Design review of the part built by this model. Coordinates are the model's own, in mm. A direction names the side the tool comes from. Give positions to 0.01 mm unless a question says otherwise; leave off trailing zeros. Write each loop counter-clockwise with the first axis right and the second up, starting at its lowest first coordinate (ties: lowest second). Pieces come first, ordered by that corner, then holes. Notation, with made-up numbers: (84.25, 13.5) -> (126.25, 13.5) arc R34 cw to (126.25, 44.5) -> close; hole circle Ø11 at (80.25, 22.5). An arc over 180 degrees is marked (long way). Write each question's results on one line, items separated by ' | '. Start each with the question number.
(1) Take a section at B-B (x = 0). State the section outline as (y, z) points, plus the area to 3 significant figures.
(2) Take a section at A-A (y = 41). State the section outline as (x, z) points.
(3) Take a section at D-D (x = -21). State the section outline as (y, z) points.
(4) Clearance check with flat-ended pins moving along their axes: pin 1 (3.5 mm diameter, centred on y = 43, z = 3, fed in from -X); pin 2 (2 mm diameter, centred on y = 9.5, z = 4.5, fed in from +X); pin 3 (3.5 mm diameter, centred on x = -5, z = 2, fed in from +Y); pin 4 (3 mm diameter, centred on y = 44.6, z = 3.5, fed in from +X). State where each tip first meets the part, or that it passes through.
(5) Take a section at C-C (z = 3.5). Count the separate pieces of the cut face and the enclosed holes in it, plus the area to 3 significant figures.
(6) For faces 5 (the face through (0, 29, 7)), 6 (the face through (5, 12, 3)), 7 (the face through (0, 34.6, 3)), 8 (the face through (-5, 13, 3)), list the 3-axis set-ups (+Z, -Z, +X, -X, +Y, -Y) from which the entire face can be reached by the end or side of a thin tool; tool diameter is ignored.
(7) Mouldability with a two-part tool opening along X and no side actions: class faces 1 (the face through (-3.924, -3.954, 3.451)), 2 (the face through (-20.1, 42, 3)), 3 (the face through (20.1, 47, 3)), 4 (the face through (0, -5, 3)) as released by +X, released by -X, zero draft, split by the parting line, or undercut.
(8) To check wall thickness, follow probe 1 along X at (y, z) = (40.5, 6); probe 2 along Y at (x, z) = (-17.5, 0.75); probe 3 along X at (y, z) = (51, 6). State the ranges of each line that lie inside material, in increasing order.
from build123d import *

# Parameters (mm, degrees)
CROQUIS1_R              = 1.65
SALIENTE_EXTRUIR1_DEPTH = 7
CORTAR_EXTRUIR1_DEPTH   = 8
CROQUIS3_R              = 2
CORTAR_EXTRUIR3_DEPTH   = 53.321320344
CROQUIS4_R              = 3.75
CORTAR_EXTRUIR4_DEPTH   = 3.121320344
CROQUIS5_R              = 3.75
CORTAR_EXTRUIR5_DEPTH   = 3.121320344


with BuildPart() as part:
    # Croquis1 → Saliente-Extruir1 (new body)
    with BuildSketch(Plane.XY):
        Polygon((-5, 27.478679656), (-5, -5), (5, -5), (5, 27.478679656), (7.121320344, 29.6), (20.102640687, 29.6), (25.1, 34.597359313), (25.1, 47.357359313), (27.221320344, 49.478679656), (27.221320344, 52.478679656), (25.1, 54.6), (20.1, 54.6), (20.1, 34.6), (-20.1, 34.6), (-20.1, 54.6), (-25.1, 54.6), (-27.221320344, 52.478679656), (-27.221320344, 49.478679656), (-25.1, 47.357359313), (-25.1, 34.597359313), (-20.102640687, 29.6), (-7.121320344, 29.6), align=None)
        Circle(CROQUIS1_R, mode=Mode.SUBTRACT)
    extrude(amount=SALIENTE_EXTRUIR1_DEPTH)

    # Croquis2 → Cortar-Extruir1 (cut, through all)
    with BuildSketch(Plane(origin=(0, 0, 0), x_dir=(-1, 0, 0), z_dir=(0, 0, -1))):
        Polygon((-5, -5), (-2.878679656, -5), (-5, -2.878679656), align=None)
        Polygon((2.878679656, -5), (5, -2.878679656), (5, -5), align=None)
    extrude(amount=-CORTAR_EXTRUIR1_DEPTH, mode=Mode.SUBTRACT)

    # Croquis3 → Cortar-Extruir3 (cut, through all)
    with BuildSketch(Plane.ZY.offset(25.1)):
        with Locations((3.5, 44.597359313)):
            Circle(CROQUIS3_R)
    extrude(amount=-CORTAR_EXTRUIR3_DEPTH, mode=Mode.SUBTRACT)

    # Croquis4 → Cortar-Extruir4 (cut, through all)
    with BuildSketch(Plane.ZY.offset(25.1)):
        with Locations((3.5, 44.597359313)):
            Circle(CROQUIS4_R)
    extrude(amount=CORTAR_EXTRUIR4_DEPTH, mode=Mode.SUBTRACT)

    # Croquis5 → Cortar-Extruir5 (cut, through all)
    with BuildSketch(Plane(origin=(25.1, 0, 0), x_dir=(0, 0, -1), z_dir=(1, 0, 0))):
        with Locations((-3.5, 44.597359313)):
            Circle(CROQUIS5_R)
    extrude(amount=CORTAR_EXTRUIR5_DEPTH, mode=Mode.SUBTRACT)


solid = part.part
Report:
1) outline: (-5, 0) -> (-1.65, 0) -> (-1.65, 7) -> (-5, 7) -> close; (1.65, 0) -> (34.6, 0) -> (34.6, 7) -> (1.65, 7) -> close | area: 254 mm2
2) outline: (-25.1, 0) -> (-20.1, 0) -> (-20.1, 7) -> (-25.1, 7) -> close; (20.1, 0) -> (25.1, 0) -> (25.1, 7) -> (20.1, 7) -> close
3) outline: (30.5, 0) -> (54.6, 0) -> (54.6, 7) -> (30.5, 7) -> close; hole circle Ø4 at (44.6, 3.5)
4) pin 1: x = -25.1 | pin 2: x = 5 | pin 3: y = 34.6 | pin 4: through
5) separate pieces: 3 | enclosed holes: 1 | area: 744 mm2
6) face 5: +Z, +X, -X, +Y, -Y | face 6: +Z, -Z, +X, -Y | face 7: +Z, -Z, +Y | face 8: +Z, -Z, -X, -Y
7) face 1: released by -X | face 2: undercut | face 3: undercut | face 4: zero draft
8) probe 1: -25.1 to -20.1, 20.1 to 25.1 | probe 2: 29.6 to 34.6 | probe 3: -27.22 to -20.1, 20.1 to 27.22
